For this review, use the dimensioned drawing (mm, ordinates from the lowest corner) and the shaded views. A direction names the side the tool comes from. Give positions to 0.01 mm unless a question says otherwise; leave off trailing zeros. Write each loop counter-clockwise with the first axis right and the second up, starting at its lowest first coordinate (ties: lowest second). Pieces come first, ordered by that corner, then holes.
1) We need section D-D on z = 37. Give the boundary of the cut face in (x, y).
2) We need section C-C on y = 46. Give the boundary of the cut face in (x, z).
3) We need section A-A on x = 31.5. Give the boundary of the cut face in (y, z).
4) Machinability: for the marked faces 1, 2 and 3, which of the approach directions +Z, -Z, +X, -X, +Y, -Y give a long, thin tool a straight path to every point of the face, cutting with its end or side? Answer none if there is none.
5) We need section B-B on z = 9. Give the boundary of the cut face in (x, y).
6) Wall thickness on line 1 along Y through (x, z) = (14.5, 25.5); line 2 along X through (y, z) = (45, 19); line 3 along Y through (x, z) = (43, 38) (1 decimal): over which ranges is each line inside the solid? List them lowest first.
7) For P1, Ø4, axis at x = 42.5, y = 69.5, coming from the +Z side; P2, Ø3, axis at x = 11.5, y = 62, coming from the +Z side (1 decimal); P3, Ø6, axis at y = 44.5, z = 29.5, coming from the -X side; P4, Ø3, axis at y = 44, z = 36, coming from the -X side, all flat-tipped, find the tip position at first contact; note any pin that passes through.
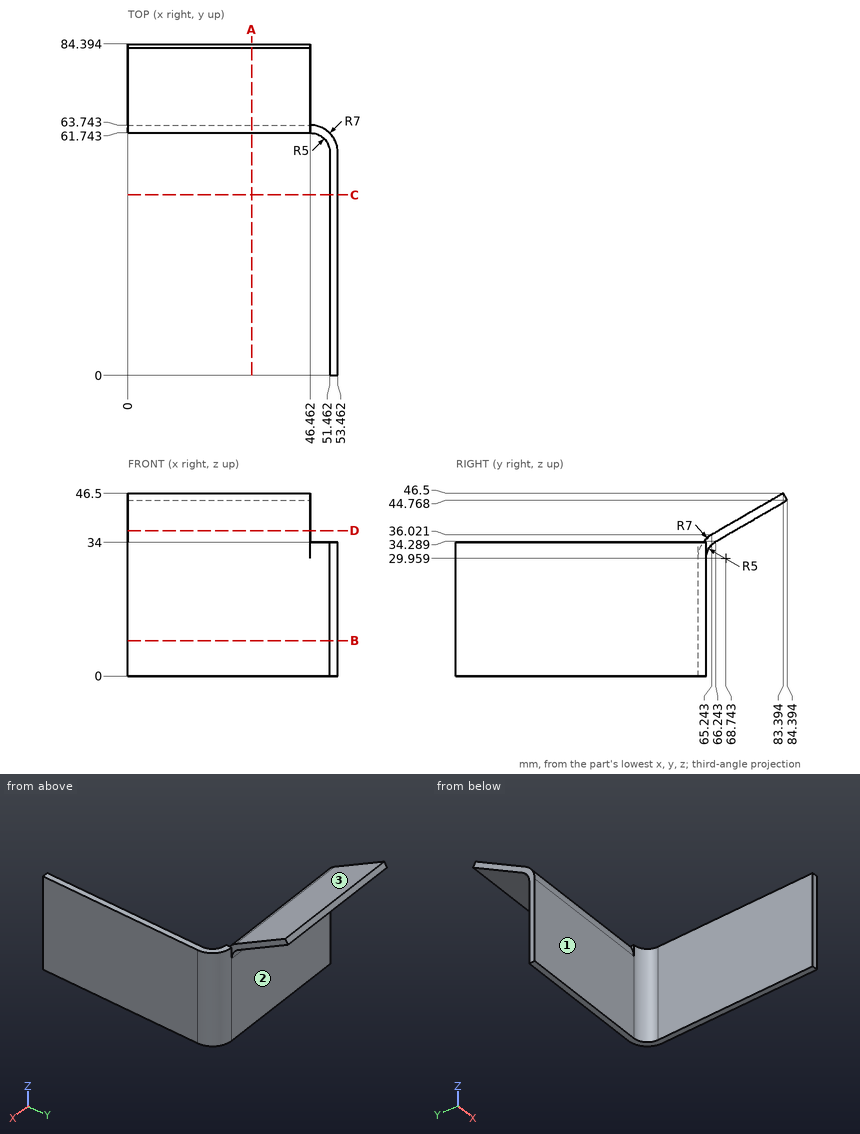
Results list:
1. outline: (0, 66.94) - (46.46, 66.94) - (46.46, 70.94) - (0, 70.94) - close
2. outline: (51.46, 0) - (53.46, 0) - (53.46, 34) - (51.46, 34) - close
3. outline: (61.74, 0) - (63.74, 0) - (63.74, 29.96) arc R5 cw to (66.24, 34.29) - (84.39, 44.77) - (83.39, 46.5) - (65.24, 36.02) arc R7 ccw to (61.74, 29.96) - close
4. face 1: +Z, -Z, -X, -Y
4. face 2: -Z, +X, -X, +Y
4. face 3: +Z, +X, -X, -Y
5. outline: (0, 61.74) - (46.46, 61.74) arc R5 cw to (51.46, 56.74) - (51.46, 0) - (53.46, 0) - (53.46, 56.74) arc R7 ccw to (46.46, 63.74) - (0, 63.74) - close
6. line 1: y = 61.74 to 63.74
6. line 2: x = 51.46 to 53.46
6. line 3: y = 68.7 to 72.7
7. P1: stops at z = 39.63
7. P2: stops at z = 34.6
7. P3: stops at x = 51.46
7. P4: passes through
